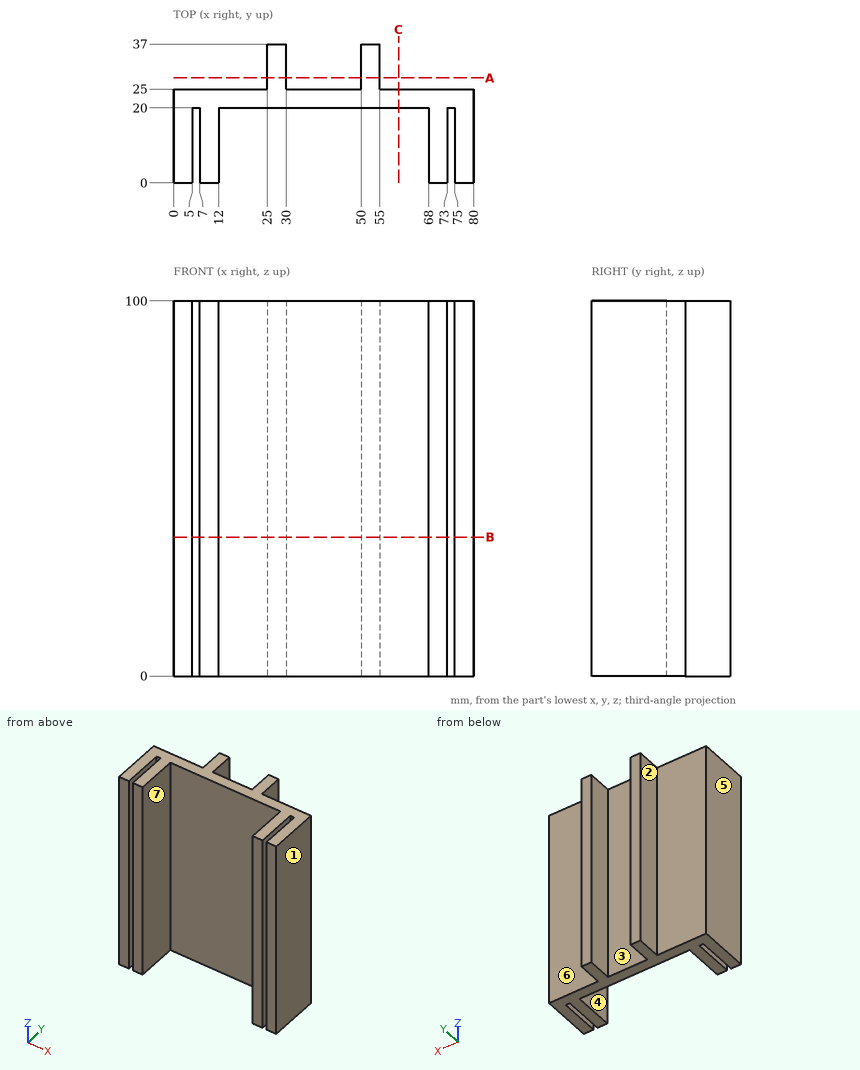
Could you check a few things on this drawing? It's one solid part, dimensions in mm from its lowest x, y, z. A direction names the side the tool comes from. Give positions to 0.01 mm unless a question says otherwise; leave off trailing zeros. Order: outer loops, then holes, each group sorted by start corner. A loop starts at its lowest first (then second) coordinate and runs counter-clockwise, first axis right, second up. Notation, with made-up numbers: (17, 13) - (66, 13) arc R10 ccw to (66, 20) - close; hole circle Ø9 at (15.25, -26). An arc over 180 degrees is marked (long way). One line per item, written item: value. Start each with the question number.
1. For P1, Ø12, axis at y = 33, z = 72.5, coming from the -X side; P2, Ø9.5, axis at y = 31, z = 29, coming from the +X side; P3, Ø1.6, axis at x = 74, z = 51.5, coming from the -Y side, each with a flat end and sliding along its axis, tell me the tip position at first contact or that it passes through.
2. Thinking about a two-plate mould opening in X: for the marked faces 5, 6 and 7, which applies, +X half, -X half, draft (parallel to the pull), parting line (faces both ways), or undercut?
3. For the marked faces 1, 2, 3 and 4, which set-ups out of +Z, -Z, +X, -X, +Y, -Y let a thin tool reach every point of the face, with its end or its side?
4. Imagine slicing it at B-B on z = 37. List the corners of the cut face in (x, y) for me, plus the area to 3 significant figures.
5. Imagine slicing it at C-C on x = 60. List the corners of the cut face in (y, z) for me, plus the area to 3 significant figures.
6. Imagine slicing it at A-A on y = 28. List the corners of the cut face in (x, z) for me, plus the area to 3 significant figures.
7. If I drill on probe 1 along X at (y, z) = (10.5, 93); probe 2 along X at (y, z) = (34.5, 88); probe 3 along Y at (x, z) = (18.5, 59), over which ranges is the centre line in solid material (lowest first)?
Values:
1. P1: x = 25
1. P2: x = 55
1. P3: y = 20
2. face 5: -X half
2. face 6: draft
2. face 7: undercut
3. face 1: +Z, -Z, +X, +Y, -Y
3. face 2: +Z, -Z, -X, +Y
3. face 3: +Z, -Z, +Y
3. face 4: +Z, -Z, -Y
4. outline: (0, 0) - (5, 0) - (5, 20) - (7, 20) - (7, 0) - (12, 0) - (12, 20) - (68, 20) - (68, 0) - (73, 0) - (73, 20) - (75, 20) - (75, 0) - (80, 0) - (80, 25) - (55, 25) - (55, 37) - (50, 37) - (50, 25) - (30, 25) - (30, 37) - (25, 37) - (25, 25) - (0, 25) - close
4. area: 920 mm²
5. outline: (20, 0) - (25, 0) - (25, 100) - (20, 100) - close
5. area: 500 mm²
6. outline: (25, 0) - (30, 0) - (30, 100) - (25, 100) - close; (50, 0) - (55, 0) - (55, 100) - (50, 100) - close
6. area: 1,000 mm²
7. probe 1: 0 to 5, 7 to 12, 68 to 73, 75 to 80
7. probe 2: 25 to 30, 50 to 55
7. probe 3: 20 to 25
